from build123d import *

# Parameters (mm, degrees)
F1_DEPTH = 10
F0_W     = 18.908922
F0_H     = 26
F2_DEPTH = 9
F4_DEPTH = 1


with BuildPart() as f1:
    # F0 (on Front) → F1 (new body)
    with BuildSketch(Plane.XZ):
        Polygon((0, -26), (0, 0), (-26, 0), (-26, -30), (0, -30), align=None)
    extrude(amount=F1_DEPTH)

    # F0 (on Front) → F2 (join)
    with BuildSketch(Plane.XZ):
        with Locations((9.454461, -13)):
            Rectangle(F0_W, F0_H)
    extrude(amount=F2_DEPTH)

    # F3 (on face) → F4 (cut)
    with BuildSketch(Plane.XZ):
        Polygon((21.377379, 0), (18.908922, 0), (18.908922, -26), (0, -26), (0, -30.423839), (21.377379, -30.423839), align=None)
    extrude(amount=F4_DEPTH, mode=Mode.SUBTRACT)


solid = f1.part
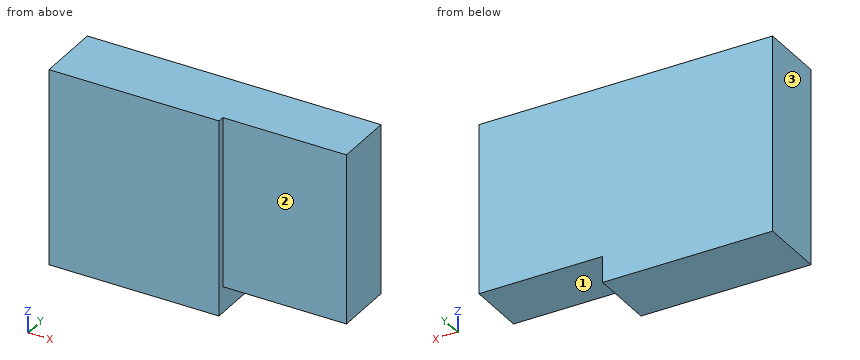
Part model, mm, in its own coordinate system. Face numbers are marked on the shaded views. A direction names the side the tool comes from. Coordinates: 2 decimals unless noted, no trailing zeros. Order: outer loops, then holes, each group sorted by start corner. A loop starts at its lowest first (then second) coordinate and runs counter-clockwise, first axis right, second up. Notation, with made-up numbers: M 69.5,58 L 81.5,58 A25 ccw 81.5,94 Z; hole C -27,3.25 d10. An arc over 180 degrees is marked long. One line per question, with ' | ' between items.
Q1. Slice it at C-C (x = 3.5). Give the cut face in (y, z), and give its area (3 significant figures).
A:
outline: M -9,-26 L 0,-26 L 0,0 L -9,0 Z | area: 234 mm^2
Q2. 3-axis set-ups, long thin cutter, end or side, ignore diameter. For the marked faces 1, 2 and 3: which of +Z, -Z, +X, -X, +Y, -Y reach the whole face in a straight line?
A:
face 1: -Z, +X, +Y, -Y | face 2: +Z, -Z, +X, -Y | face 3: +Z, -Z, -X, +Y, -Y
Q3. Slice it at B-B (z = -6). Give the cut face in (x, y).
A:
outline: M -26,-10 L 0,-10 L 0,-9 L 18.91,-9 L 18.91,0 L -26,0 Z
Q4. Slice it at A-A (y = -4.25). Give the cut face in (x, z).
A:
outline: M -26,-30 L 0,-30 L 0,-26 L 18.91,-26 L 18.91,0 L -26,0 Z
Q5. Drill centre lines: line 1 (Z direction, x = 9, y = -0.5); line 2 (Y direction, x = 11.5, z = -23.75). Where is each one in solid material? Low to high.
A:
line 1: z = -26 to 0 | line 2: y = -9 to 0
Q6. Pin check, flat tip, straight feed: P1, Ø5.5, axis at x = 5, z = -11, coming from the -Y side. Stop position of the tip, or through.
A:
P1: stops at y = -9
